Here's how the part is built. I have some questions about the finished solid (model axes, mm). A direction names the side the tool comes from. Coordinates: 2 decimals unless noted, no trailing zeros. Loops run counter-clockwise (first coordinate to the right, second up) from the corner with the lowest first, then second, coordinate; pieces in that order, holes last. Notation, with made-up numbers: (-20.5, 65.5) -> (-13.5, 65.5) arc R22 cw to (-13.5, 99.5) -> close; hole circle Ø11 at (82.5, 66.5). An arc over 180 degrees is marked (long way). Answer as a JSON object with one key per item and string values. Group by question number.
1) I need wall thicknesses on probe 1 along Y at (x, z) = (-2, 0.85); probe 2 along X at (y, z) = (14, 2.45); probe 3 along Y at (x, z) = (3, 0.65). Which ranges of each line are inside material? Lowest first, please. Write a range as [from, to].
2) I want a section at C-C (y = 13.5). Write out the boundary of the cut face in (x, z).
3) Which directions (+Z, -Z, +X, -X, +Y, -Y) give clear straight access to the entire face, cutting with the end or side of a thin tool? Please do faces 1 (the flat face through (0, -16, 1)), 2 (the flat face through (-1.65, 20.5, 1.5)), 3 (the flat face through (12.5, -23, 1)), 4 (the cylindrical face through (13.424, -9.765, 1.479)).
4) I'm going to push flat-ended pins straight in: pin 1 (5 mm diameter, centred on x = 12, y = 12, fed in from -Z); pin 2 (0.9 mm diameter, centred on y = 24, z = 1, fed in from -X); pin 3 (0.9 mm diameter, centred on y = -22, z = 1.5, fed in from +X); pin 4 (1.5 mm diameter, centred on x = -4, z = 2, fed in from -Y). Where does each tip first touch, or does it pass through?
5) If we mould it in two halves opening along X, with no side actions, what happens to faces 5 (the flat face through (-10, -25, 1)), 6 (the flat face through (12.5, 23, 1)), 7 (the flat face through (1.65, -20.5, 1.5)), 8 (the flat face through (-1.65, -20.5, 1.5))? For each: +X half, -X half, draft (parallel to the pull), parting line (faces both ways), or undercut.
6) I want a section at B-B (x = -6). Write out the boundary of the cut face in (y, z).
7) I want a section at D-D (x = 13.5). Write out the boundary of the cut face in (y, z), then the cut area to 3 significant figures.
8) I want a section at A-A (y = 0). Write out the boundary of the cut face in (x, z), then the cut area to 3 significant figures.
```python
from build123d import *

# Parameters (mm, degrees)
SKETCH_1_R      = 6.65
SKETCH_1_R_2    = 2.65
EXTRUDE_1_DEPTH = 3


with BuildPart() as part:
    # 草图1 → 凸台-拉伸1 (new body)
    with BuildSketch(Plane.XY):
        with BuildLine():
            Line((17.5, -21), (17.5, 21))
            Line((17.5, 21), (12.5, 21))
            Line((12.5, 21), (12.5, 25))
            Line((12.5, 25), (7.5, 25))
            Line((7.5, 25), (7.5, 21))
            Line((7.5, 21), (1.65, 21))
            Line((1.65, 21), (1.65, 20))
            ThreePointArc((1.65, 20), (3.806776436, 18.5), (1.65, 17))
            Line((1.65, 17), (1.65, 16))
            Line((1.65, 16), (-1.65, 16))
            Line((-1.65, 16), (-1.65, 17))
            ThreePointArc((-1.65, 17), (-3.806776436, 18.5), (-1.65, 20))
            Line((-1.65, 20), (-1.65, 21))
            Line((-1.65, 21), (-7.5, 21))
            Line((-7.5, 21), (-7.5, 25))
            Line((-7.5, 25), (-12.5, 25))
            Line((-12.5, 25), (-12.5, 21))
            Line((-12.5, 21), (-17.5, 21))
            Line((-17.5, 21), (-17.5, -21))
            Line((-17.5, -21), (-12.5, -21))
            Line((-12.5, -21), (-12.5, -25))
            Line((-12.5, -25), (-7.5, -25))
            Line((-7.5, -25), (-7.5, -21))
            Line((-7.5, -21), (-1.65, -21))
            Line((-1.65, -21), (-1.65, -20))
            ThreePointArc((-1.65, -20), (-3.806776436, -18.5), (-1.65, -17))
            Line((-1.65, -17), (-1.65, -16))
            Line((-1.65, -16), (1.65, -16))
            Line((1.65, -16), (1.65, -17))
            ThreePointArc((1.65, -17), (3.806776436, -18.5), (1.65, -20))
            Line((1.65, -20), (1.65, -21))
            Line((1.65, -21), (7.5, -21))
            Line((7.5, -21), (7.5, -25))
            Line((7.5, -25), (12.5, -25))
            Line((12.5, -25), (12.5, -21))
            Line((12.5, -21), (17.5, -21))
        make_face()
        Circle(SKETCH_1_R, mode=Mode.SUBTRACT)
        with Locations((11.999602077, -11.999602077)):
            Circle(SKETCH_1_R_2, mode=Mode.SUBTRACT)
        with Locations((-11.999602077, -11.999602077)):
            Circle(SKETCH_1_R_2, mode=Mode.SUBTRACT)
        with Locations((-11.999602077, 11.999602077)):
            Circle(SKETCH_1_R_2, mode=Mode.SUBTRACT)
        with Locations((11.999602077, 11.999602077)):
            Circle(SKETCH_1_R_2, mode=Mode.SUBTRACT)
    extrude(amount=EXTRUDE_1_DEPTH)


solid = part.part
```
Determined:
{
 "1": {"probe 1": "[-21, -20.09], [-16.91, -6.34], [6.34, 16.91], [20.09, 21]", "probe 2": "[-17.5, -13.74], [-10.26, 10.26], [13.74, 17.5]", "probe 3": "[-21, -19.89], [-17.11, -5.93], [5.93, 17.11], [19.89, 21]"},
 "2": {"outline": "(-17.5, 0) -> (-14.18, 0) -> (-14.18, 3) -> (-17.5, 3) -> close; (-9.82, 0) -> (9.82, 0) -> (9.82, 3) -> (-9.82, 3) -> close; (14.18, 0) -> (17.5, 0) -> (17.5, 3) -> (14.18, 3) -> close"},
 "3": {"face 1": "+Z, -Z, -Y", "face 2": "+Z, -Z, +Y", "face 3": "+Z, -Z, +X, -Y", "face 4": "+Z, -Z"},
 "4": {"pin 1": "through", "pin 2": "x = -12.5", "pin 3": "x = 12.5", "pin 4": "y = -21"},
 "5": {"face 5": "draft", "face 6": "+X half", "face 7": "undercut", "face 8": "undercut"},
 "6": {"outline": "(-21, 0) -> (-2.87, 0) -> (-2.87, 3) -> (-21, 3) -> close; (2.87, 0) -> (21, 0) -> (21, 3) -> (2.87, 3) -> close"},
 "7": {"outline": "(-21, 0) -> (-14.18, 0) -> (-14.18, 3) -> (-21, 3) -> close; (-9.82, 0) -> (9.82, 0) -> (9.82, 3) -> (-9.82, 3) -> close; (14.18, 0) -> (21, 0) -> (21, 3) -> (14.18, 3) -> close", "area": "99.8 mm^2"},
 "8": {"outline": "(-17.5, 0) -> (-6.65, 0) -> (-6.65, 3) -> (-17.5, 3) -> close; (6.65, 0) -> (17.5, 0) -> (17.5, 3) -> (6.65, 3) -> close", "area": "65.1 mm^2"}
}
